Geometry: see drawing. Coordinates: mm, zero at the bounding-box minimum. Give positions to 0.01 mm unless a question says otherwise; leave off trailing zeros. Write each loop counter-clockwise with the first axis right and the second up, starting at its lowest first coordinate (ties: lowest second). Pieces come first, ordered by that corner, then holes. Notation, with made-up numbers: (74, -34.75) - (119, -34.75) arc R29 cw to (119, -9.75) - close; hole circle Ø7 at (56, 26.5). An arc over 180 degrees is marked (long way). Return JSON: item names as keys, results as strings.
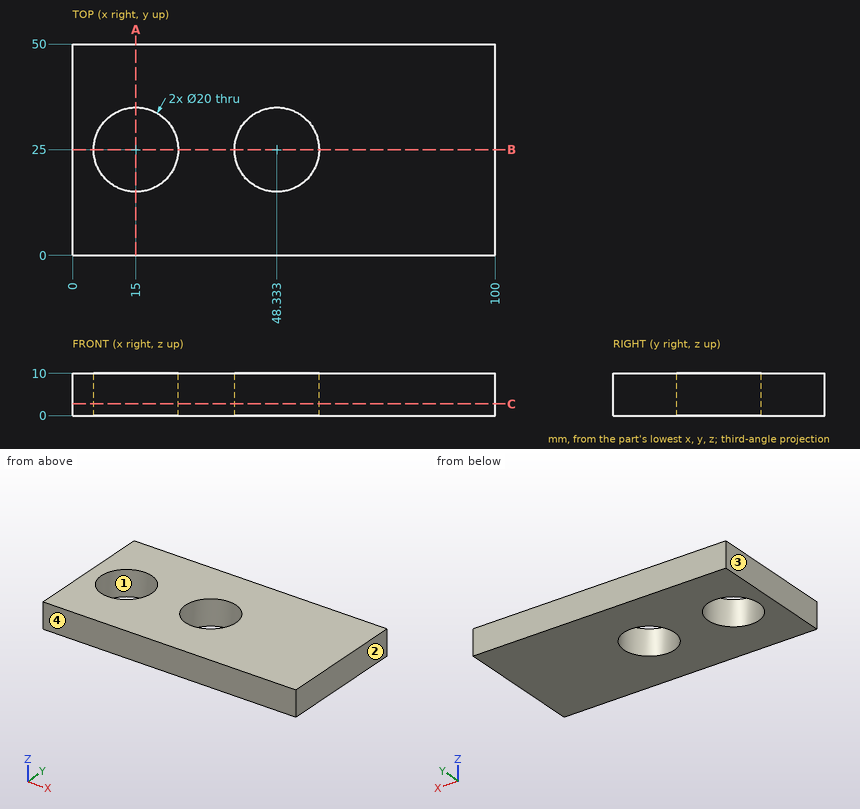
Q1. Section query A-A, the plane x = 15. Return the cut outline in (y, z), plus the area to 3 significant figures.
Answer key:
{"outline": "(0, 0) - (15, 0) - (15, 10) - (0, 10) - close; (35, 0) - (50, 0) - (50, 10) - (35, 10) - close", "area": "300 mm^2"}
Q2. Section query C-C, the plane z = 2.75. Return the cut outline in (x, y), plus the area to 3 significant figures.
Answer key:
{"outline": "(0, 0) - (100, 0) - (100, 50) - (0, 50) - close; hole circle Ø20 at (15, 25); hole circle Ø20 at (48.33, 25)", "area": "4,370 mm^2"}
Q3. Section query B-B, the plane y = 25. Return the cut outline in (x, z).
Answer key:
{"outline": "(0, 0) - (5, 0) - (5, 10) - (0, 10) - close; (25, 0) - (38.33, 0) - (38.33, 10) - (25, 10) - close; (58.33, 0) - (100, 0) - (100, 10) - (58.33, 10) - close"}
Q4. Mould query, pull axis X, two halves, no side actions, for the marked faces 1, 2, 3 and 4. Classes: pulls with the +X half, pulls with the -X half, needs draft (parallel to the pull), parting line crosses it, or undercut.
Answer key:
{"face 1": "undercut", "face 2": "pulls with the +X half", "face 3": "pulls with the -X half", "face 4": "needs draft"}
Q5. Material intervals for probe 1 along X at (y, z) = (25, 3.75); probe 2 along Y at (x, z) = (15, 5.25); probe 3 along X at (y, z) = (17.5, 3) (1 decimal), sorted ascending. Write a range as [from, to].
Answer key:
{"probe 1": "x = [0, 5], [25, 38.33], [58.33, 100]", "probe 2": "y = [0, 15], [35, 50]", "probe 3": "x = [0, 8.4], [21.6, 41.7], [54.9, 100]"}
